Check sheet for the drawn part. Datum: minimum x, y, z corner. Units: mm. Coordinates: 2 decimals unless noted, no trailing zeros. Write each loop counter-clockwise with the first axis right and the second up, starting at its lowest first coordinate (ties: lowest second). Pieces come first, ordered by that corner, then holes. Notation, with made-up numbers: (11.5, 33.25) - (35.5, 33.25) arc R15 cw to (35.5, 51.25) - close; hole circle Ø5 at (76, 26.5). An arc over 180 degrees is marked (long way). Answer as CSV lines item,"result". Start each with the question number.
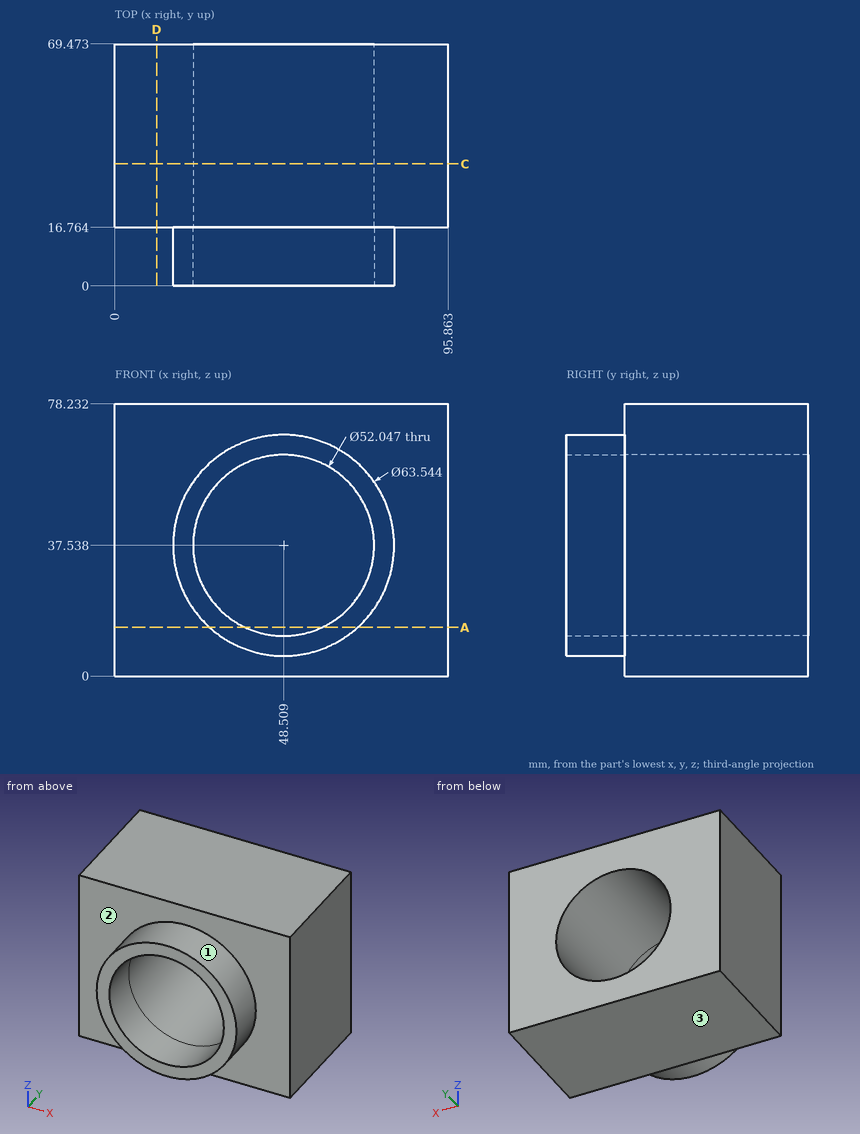
(1) Material ranges on probe 1 along Y at (x, z) = (9.5, 7); probe 2 along Z at (x, y) = (59, 13.5); probe 3 along Z at (x, y) = (62, 50) (1 decimal), recorded low to high. Write a range as from..to.
(2) Cross-section at A-A on z = 14. Record the boundary of the cut face in (x, y), plus the area to 3 significant figures.
(3) Cross-section at C-C on y = 35. Record the boundary of the cut face in (x, z).
(4) Cross-section at D-D on x = 12. Record the boundary of the cut face in (y, z).
(5) Release check for a two-part mould opening along Z. For the marked faces 1, 2 and 3 record: pulls with the +Z half, pulls with the -Z half, needs draft (parallel to the pull), parting line crosses it, or undercut.
(6) Go/stop test with flat-tipped pins: P1, Ø6, axis at x = 10.5, z = 61, coming from the -Y side; P2, Ø2, axis at x = 29, z = 53, coming from the +Y side; P3, Ø1.5, axis at y = 15.5, z = 54.5, coming from the -X side (1 decimal); P4, Ø5, axis at x = 59.5, y = 8, coming from the +Z side. Record where each tip stops, or that it passes through.
Checked values:
1,probe 1,"16.76..69.47"
1,probe 2,"7.55..13.72, 61.35..67.53"
1,probe 3,"0..15.3, 59.8..78.2"
2,outline,"(0, 16.76) - (27.17, 16.76) - (27.17, 0) - (37.41, 0) - (37.41, 69.47) - (0, 69.47) - close; (59.61, 0) - (69.85, 0) - (69.85, 16.76) - (95.86, 16.76) - (95.86, 69.47) - (59.61, 69.47) - close"
2,area,"4,230 mm^2"
3,outline,"(0, 0) - (95.86, 0) - (95.86, 78.23) - (0, 78.23) - close; hole circle Ø52.05 at (48.51, 37.54)"
4,outline,"(16.76, 0) - (69.47, 0) - (69.47, 78.23) - (16.76, 78.23) - close"
5,face 1,"parting line crosses it"
5,face 2,"needs draft"
5,face 3,"pulls with the -Z half"
6,P1,"y = 16.76"
6,P2,"through"
6,P3,"x = 21.2"
6,P4,"z = 68.15"
